```python
from build123d import *

# Parameters (mm, degrees)
SKETCH2_W           = 19
SKETCH2_H           = 14
BOSS_EXTRUDE1_DEPTH = 9
SKETCH3_W           = 15
SKETCH3_H           = 5
CUT_EXTRUDE1_DEPTH  = 5
SKETCH6_W           = 15
SKETCH6_H           = 7
CUT_EXTRUDE3_DEPTH  = 4
SKETCH7_W           = 15
SKETCH7_H           = 5
CUT_EXTRUDE4_DEPTH  = 4


with BuildPart() as part:
    # Sketch2 → Boss-Extrude1 (new body)
    with BuildSketch(Plane.XY):
        Rectangle(SKETCH2_W, SKETCH2_H)
    extrude(amount=BOSS_EXTRUDE1_DEPTH)

    # Sketch3 → Cut-Extrude1 (cut)
    with BuildSketch(Plane.XY.offset(9)):
        with Locations((0, -2.5)):
            Rectangle(SKETCH3_W, SKETCH3_H)
    extrude(amount=-CUT_EXTRUDE1_DEPTH, mode=Mode.SUBTRACT)

    # Sketch6 → Cut-Extrude3 (cut)
    with BuildSketch(Plane(origin=(0, 7, 0), x_dir=(1, 0, 0), z_dir=(0, 1, 0))):
        with Locations((0, -3.5)):
            Rectangle(SKETCH6_W, SKETCH6_H)
    extrude(amount=-CUT_EXTRUDE3_DEPTH, mode=Mode.SUBTRACT)

    # Sketch7 → Cut-Extrude4 (cut)
    with BuildSketch(Plane(origin=(0, 3, 0), x_dir=(1, 0, 0), z_dir=(0, 1, 0))):
        with Locations((0, -4.5)):
            Rectangle(SKETCH7_W, SKETCH7_H)
    extrude(amount=-CUT_EXTRUDE4_DEPTH, mode=Mode.SUBTRACT)


solid = part.part
```
The listing builds one solid part. Answer for the finished solid, in the listing's coordinates (mm). A direction names the side the tool comes from. Coordinates: 2 decimals unless noted, no trailing zeros. Write each loop counter-clockwise with the first axis right and the second up, starting at its lowest first coordinate (ties: lowest second). Pieces come first, ordered by that corner, then holes. Notation, with made-up numbers: M 76,68 L 98,68 A22 ccw 98,106 Z; hole C 18,-35.75 d3. An arc over 180 degrees is marked long. Use a Markdown table: item, result. Add a question column.
1. Section D-D (y = 5.5) is taken. Give the vertices of the cut face in (x, z).
2. Section C-C (z = 3) is taken. Give the vertices of the cut face in (x, y).
3. Section B-B (y = 0.5) is taken. Give the vertices of the cut face in (x, z).
4. Given P1, Ø1.2, axis at x = -0.5, y = -2.5, coming from the +Z side; P2, Ø2.5, axis at x = -0.5, z = 5.5, coming from the +Y side; P3, Ø1.6, axis at x = 3.5, z = 3.5, coming from the +Y side, each flat-ended and moving along its own axis, determine where each tip first touches the part or whether it passes through.
5. Section A-A (x = 5) is taken. Give the vertices of the cut face in (y, z).
6. Which of the six approach directions +Z, -Z, +X, -X, +Y, -Y give full straight-line access (tool end or side, diameter ignored) to faces 4 (the flat face through (0, -1, 3)), 5 (the flat face through (0, 1, 2)), 6 (the flat face through (0, -5, 7))?
7. Straight lines are drawn through the part: line 1 along X through (y, z) = (3, 6); line 2 along Z through (x, y) = (-0.25, 1.5); line 3 along Y through (x, z) = (2, 7.75). For each, find the intervals that lie inside material, in ascending order. Write a range as [from, to].
8. For a pull along Z with two mould halves and no side action, classify faces 1 (the flat face through (-9.5, 0, 4)), 2 (the flat face through (0, -3, 4)), 3 (the flat face through (0, 4, 7)) as +Z half, -Z half, draft (parallel to the pull), parting line (faces both ways), or undercut.
Data:
| question | item | result |
|---|---|---|
| 1 | outline | M -9.5,0 L -7.5,0 L -7.5,7 L 7.5,7 L 7.5,0 L 9.5,0 L 9.5,9 L -9.5,9 Z |
| 2 | outline | M -9.5,-7 L 9.5,-7 L 9.5,7 L 7.5,7 L 7.5,-1 L -7.5,-1 L -7.5,7 L -9.5,7 Z |
| 3 | outline | M -9.5,0 L 9.5,0 L 9.5,9 L -9.5,9 Z; hole M -7.5,2 L 7.5,2 L 7.5,7 L -7.5,7 Z |
| 4 | P1 | stops at z = 4 |
| 4 | P2 | stops at y = -5 |
| 4 | P3 | stops at y = -1 |
| 5 | outline | M -7,0 L 3,0 L 3,2 L -1,2 L -1,4 L -5,4 L -5,9 L -7,9 Z; M 0,7 L 7,7 L 7,9 L 0,9 Z |
| 6 | face 4 | +Z, +Y |
| 6 | face 5 | +Y |
| 6 | face 6 | +Z |
| 7 | line 1 | x = [-9.5, -7.5], [7.5, 9.5] |
| 7 | line 2 | z = [0, 2], [7, 9] |
| 7 | line 3 | y = [-7, -5], [0, 7] |
| 8 | face 1 | draft |
| 8 | face 2 | +Z half |
| 8 | face 3 | undercut |
